Here's how the part is built. I have some questions about the finished solid (model axes, mm). A direction names the side the tool comes from. Give positions to 0.01 mm unless a question says otherwise; leave off trailing zeros. Loops run counter-clockwise (first coordinate to the right, second up) from the corner with the lowest first, then second, coordinate; pieces in that order, holes last.
Q1. We'd pull the mould along Z, two halves only. Please class faces 6 (the face through (44, 3, -81.5)), 7 (the face through (-2.578, 6.338, 2.493)), 8 (the face through (43.48, -8.31, -97.81)): +Z half, -Z half, draft (parallel to the pull), parting line (faces both ways), or undercut.
Q2. If we section it at C-C (z = -32): Please give me the cut outline in (x, y).
Q3. Will these pins go through, and if not, where does the flat tip stop? P1, Ø2.5, axis at y = 13.95, z = -97, coming from the +X side; P2, Ø5.5, axis at x = 0, y = 6, coming from the +Z side; P3, Ø4.5, axis at x = 0, y = 6, coming from the +Z side; P4, Ø6, axis at x = 31, y = -10.5, coming from the -Z side.
Q4. If we section it at B-B (y = 6): Please give me the cut outline in (x, z).
Q5. I need wall thicknesses on line 1 (X direction, y = 0, z = 2.45); line 2 (X direction, y = 0, z = 0.8); line 3 (Y direction, x = 44, z = -97). Which ranges of each line are inside material? Lowest first, please.
Q6. If we section it at A-A (x = 0): Please give me the cut outline in (y, z), plus the area to 3 significant figures.
Q7. For faces 1 (the face through (43.48, 12.69, -97.81)), 2 (the face through (43, -10, -27)), 3 (the face through (3.422, 0.338, 2.493)), 4 (the face through (10, -11, 0)), 5 (the face through (43, 17, -91)), which set-ups out of +Z, -Z, +X, -X, +Y, -Y let a thin tool reach every point of the face, with its end or its side?
Q8. If we section it at D-D (y = -16): Please give me the cut outline in (x, z).
Autodesk Inventor part; units mm, degrees
ref_plane "YZ Plane" through (0, 0, 0) normal (1, 0, 0) x (0, 1, 0)
ref_plane "XZ Plane" through (0, 0, 0) normal (0, 1, 0) x (-1, 0, 0)
ref_plane "XY Plane" through (0, 0, 0) normal (0, 0, 1) x (1, 0, 0)
sketch "Sketch1" plane through (0, 0, 0) normal (0, 0, 1) x (1, 0, 0)
  arc A0 (10, 0) -> (-10, 0) centre (0, 0) ccw
  line L0 (-10, 0) -> (-10, -20)
  line L1 (-10, -20) -> (10, -20)
  line L2 (10, -10) -> (10, 0)
  line L3 (10, -20) -> (45, -20)
  line L4 (45, -20) -> (45, -10)
  line L5 (45, -10) -> (10, -10)
  dimension "d1" = 20
  dimension "d2" = 35
  dimension "d3" = 10
extrude "Extrusion1" add sketch "Sketch1" along normal blind 3
sketch "Sketch2" plane through (0, 0, 0) normal (0, 0, -1) x (-1, 0, 0)
  line L0 (10, -20) -> (-45, -20)
  line L1 (-45, -10) -> (-10, -10)
  line L2 (-45, -20) -> (-42, -20)
  line L3 (-42, -20) -> (-42, -10)
  line L4 (-42, -10) -> (-45, -10)
  line L5 (-45, -10) -> (-45, -20)
  point P0 (0, 0)
  dimension "d6" = 3
extrude "Extrusion2" add sketch "Sketch2" along normal blind 100
sketch "Sketch3" plane through (45, -20, 3) normal (1, 0, 0) x (0, 0, -1)
  point P0 (3, 20)
sketch "Sketch4" plane through (45, -20, 3) normal (1, 0, 0) x (0, 0, -1)
  point P0 (3, 20)
sketch "Sketch5" plane through (10, -10, 3) normal (0, 1, 0) x (1, 0, 0)
  line L0 (32, 3) -> (32, 103)
  line L1 (32, 103) -> (35, 103)
  line L2 (35, 103) -> (35, 84.5)
  line L3 (35, 84.5) -> (32, 84.5)
  line L4 (32, 84.5) -> (32, 103)
  point P0 (-10, 3)
  dimension "d9" = 3
  dimension "d10" = 18.5
extrude "Extrusion3" add sketch "Sketch5" along normal blind 27
sketch "Sketch6" plane through (0, 0, 3) normal (0, 0, 1) x (1, 0, 0)
  point P0 (0, 0)
  point P1 (0, 6)
  point P2 (0, -6)
  point P3 (6, 0)
  point P4 (-6, 0)
hole "Hole1" at (0, 6, 3) at (0, -6, 3) at (6, 0, 3) at (-6, 0, 3) direction (0, 0, -1) diameter 4.2 end through all counterbore diameter 5.2 counterbore depth 1
sketch "Sketch7" plane through (45, -20, 3) normal (1, 0, 0) x (0, 0, -1)
  line L0 (103, 0) -> (103, 37)
  point P0 (3, 20)
  point P1 (100, 12.9534)
  point P2 (100, 33.9534)
  point P3 (87.5, 12.9534)
  point P4 (87.5, 33.9534)
hole "Hole2" at (45, -7.0466, -97) at (45, 13.9534, -97) at (45, -7.0466, -84.5) at (45, 13.9534, -84.5) direction (-1, 0, 0) diameter 3 end through all
properties part number "Cam_mount"
Check sheet entries:
1. face 6: +Z half
1. face 7: draft
1. face 8: undercut
2. outline: (42, -20) - (45, -20) - (45, -10) - (42, -10) - close
3. P1: passes through
3. P2: stops at z = 3
3. P3: stops at z = 2
3. P4: stops at z = 0
4. outline: (-8, 0) - (-2.1, 0) - (-2.1, 2) - (-2.6, 2) - (-2.6, 3) - (-8, 3) - close; (2.1, 0) - (8, 0) - (8, 3) - (2.6, 3) - (2.6, 2) - (2.1, 2) - close; (42, -100) - (45, -100) - (45, -81.5) - (42, -81.5) - close
5. line 1: x = -10 to -8.6, -3.4 to 3.4, 8.6 to 10
5. line 2: x = -10 to -8.1, -3.9 to 3.9, 8.1 to 10
5. line 3: y = -20 to -8.55, -5.55 to 12.45, 15.45 to 17
6. outline: (-20, 0) - (-8.1, 0) - (-8.1, 2) - (-8.6, 2) - (-8.6, 3) - (-20, 3) - close; (-3.9, 0) - (3.9, 0) - (3.9, 2) - (3.4, 2) - (3.4, 3) - (-3.4, 3) - (-3.4, 2) - (-3.9, 2) - close; (8.1, 0) - (10, 0) - (10, 3) - (8.6, 3) - (8.6, 2) - (8.1, 2) - close
6. area: 62.8 mm2
7. face 1: +X, -X
7. face 2: +Z, +X, +Y
7. face 3: +Z
7. face 4: -Z, -X, +Y, -Y
7. face 5: +Z, -Z, +X, -X, +Y
8. outline: (-10, 0) - (42, 0) - (42, -100) - (45, -100) - (45, 3) - (-10, 3) - close
